Source: CAD feature listing. Evaluate the final solid. Frame: model axes, mm. A direction names the side the tool comes from. Round coordinates to 2 decimals unless told otherwise and drop trailing zeros. Order: outer loops, then holes, each group sorted by start corner. A loop starts at its lowest first (then second) coordinate and runs counter-clockwise, first axis right, second up. Notation, with made-up numbers: M -32.5,68 L -18.5,68 A11 ccw -18.5,81 Z; hole C 0.5,-37 d9. An arc over 180 degrees is marked long. Use CSV: the item, a comma, the result in double quotes. Start each with the question number.
```python
from build123d import *

# Parameters (mm, degrees)
SKETCH_2_R          = 21
CUT_EXTRUDE_1_DEPTH = 39.418745425
SKETCH_3_W          = 3.44
SKETCH_3_H          = 16
CHAMFER_1_SIZE      = 0.42


with BuildPart() as part:
    # 草图1 → 旋转1 (revolve)
    with BuildSketch(Plane.XY, mode=Mode.PRIVATE) as revolve_1_sk:
        with BuildLine():
            Line((0, 0), (-10.5, 0))
            Line((-10.5, 0), (-10.5, 15.6))
            ThreePointArc((-10.5, 15.6), (-15.293686607, 16.575499043), (-20, 17.910281389))
            Line((-20, 17.910281389), (-20, 22.473460386))
            ThreePointArc((-20, 22.473460386), (-10.154266119, 25.111616828), (0, 26))
            Line((0, 26), (0, 0))
        make_face()
    revolve(revolve_1_sk.sketch.rotate(Axis((0, 26, 0), (0, -1, 0)), 270), axis=Axis((0, 26, 0), (0, -1, 0)))

    # 草图2 → 切除-拉伸1 (cut, through all)
    with BuildSketch(Plane(origin=(0, 0, 0), x_dir=(1, 0, 0), z_dir=(0, 1, 0))):
        Circle(SKETCH_2_R)
        with BuildLine():
            ThreePointArc((4.524283339, 16.696844937), (0, 20), (-4.524283339, 16.696844937))
            ThreePointArc((-4.524283339, 16.696844937), (-8.31833689, 11.449208504), (-14.48156274, 9.462457989))
            ThreePointArc((-14.48156274, 9.462457989), (-19.021130326, 6.180339887), (-17.277723618, 0.856759687))
            ThreePointArc((-17.277723618, 0.856759687), (-13.459351819, -4.373208504), (-13.474381322, -10.848724283))
            ThreePointArc((-13.474381322, -10.848724283), (-11.755705046, -16.180339887), (-6.153937105, -16.16733833))
            ThreePointArc((-6.153937105, -16.16733833), (0, -14.152), (6.153937105, -16.16733833))
            ThreePointArc((6.153937105, -16.16733833), (11.755705046, -16.180339887), (13.474381322, -10.848724283))
            ThreePointArc((13.474381322, -10.848724283), (13.459351819, -4.373208504), (17.277723618, 0.856759687))
            ThreePointArc((17.277723618, 0.856759687), (19.021130326, 6.180339887), (14.48156274, 9.462457989))
            ThreePointArc((14.48156274, 9.462457989), (8.31833689, 11.449208504), (4.524283339, 16.696844937))
        make_face(mode=Mode.SUBTRACT)
    extrude(amount=CUT_EXTRUDE_1_DEPTH, mode=Mode.SUBTRACT)

    # 草图3 → 切除-旋转1 (revolve, cut)
    with BuildSketch(Plane.XY, mode=Mode.PRIVATE) as cut_revolve_1_sk:
        with Locations((1.72, 8)):
            Rectangle(SKETCH_3_W, SKETCH_3_H)
    revolve(cut_revolve_1_sk.sketch.rotate(Axis((0, 0, 0), (0, 1, 0)), 90), axis=Axis((0, 0, 0), (0, 1, 0)), mode=Mode.SUBTRACT)

    # 倒角1
    chamfer_1_edges = [part.edges().sort_by_distance(p)[0] for p in [
        (0, 0, -10.5),
    ]]
    chamfer(chamfer_1_edges, length=CHAMFER_1_SIZE)


solid = part.part
```
(1) Reachability of faces 4 (the face through (13.43, 20.23, 4.46)), 5 (the face through (-1.033, 8.112, -3.281)) from +Z, -Z, +X, -X, +Y, -Y: full face, straight path, thin tool, end or side. Return the list, or none.
(2) Section C-C on x = 0. Return loops of the section in (y, z).
(3) Contact query for flat-ended pins moving along their axis: P1, Ø4, axis at x = -5, z = -6.5, coming from the +Y side; P2, Ø3, axis at x = 14.5, y = 13, coming from the -Z side; P3, Ø5, axis at x = 5, y = 11, coming from the -Z side; P4, Ø8, axis at x = 12.5, y = 14.5, coming from the +Z side. Output: stop coordinate, or through.
(4) Section D-D on y = 19.5. Return loops of the section in (x, z).
(5) Section A-A on y = 2. Return loops of the section in (x, z), plus the area to 3 significant figures.
(6) Line query: line 1 along X through (y, z) = (12.75, 0); line 2 along Z through (x, y) = (0.5, 9.5); line 3 along Y through (x, z) = (-13, -7.5). Output: solid intervals per line, ascending.
(7) Draft query along Z for faces 1 (the face through (0, 20, -20)), 2 (the face through (11.687, 20.196, 16.229)), 3 (the face through (-3.2, 8.1, 10)). Return one class per face: pulls with the +Z half, pulls with the -Z half, needs draft (parallel to the pull), parting line crosses it, or undercut.
(8) Section B-B on z = 0. Return loops of the section in (x, y).
Results below:
1,face 4,"+X, +Y, -Y"
1,face 5,"-Y"
2,outline,"M 0,-10.08 L 0.42,-10.5 L 15.6,-10.5 A64.72 ccw 17.91,-20 L 22.47,-20 A58.48 ccw 24.26,14.15 L 16.31,14.15 A64.72 ccw 15.6,10.5 L 0.42,10.5 L 0,10.08 L 0,3.44 L 16,3.44 L 16,-3.44 L 0,-3.44 Z"
3,P1,"stops at y = 25.67"
3,P2,"passes through"
3,P3,"stops at z = -10.2"
3,P4,"stops at z = 16.9"
4,outline,"M -17.28,-0.86 A4.75 ccw -14.48,-9.46 A10.4 cw -4.52,-16.7 A4.75 ccw 4.52,-16.7 A10.4 cw 14.48,-9.46 A4.75 ccw 17.28,-0.86 A10.4 cw 13.47,10.85 A4.75 ccw 6.15,16.17 A10.4 cw -6.15,16.17 A4.75 ccw -13.47,10.85 A10.4 cw Z"
5,outline,"C 0,0 d21; hole C 0,0 d6.88"
5,area,"309 mm2"
6,line 1,"x = -10.5 to -3.44, 3.44 to 10.5"
6,line 2,"z = -10.49 to -3.4, 3.4 to 10.49"
6,line 3,"y = 16.51 to 24.04"
7,face 1,"pulls with the -Z half"
7,face 2,"undercut"
7,face 3,"parting line crosses it"
8,outline,"M -16.24,16.81 A64.72 ccw -10.5,15.6 L -10.5,0.42 L -10.08,0 L -3.44,0 L -3.44,16 L 3.44,16 L 3.44,0 L 10.08,0 L 10.5,0.42 L 10.5,15.6 A64.72 ccw 16.24,16.81 L 16.24,23.7 A58.48 ccw -16.24,23.7 Z"
